Check sheet for the modelled part. Datum: model origin and axes. Units: mm. Face numbers are marked on the shaded views. A direction names the side the tool comes from. Coordinates: 2 decimals unless noted, no trailing zeros. Order: outer loops, then holes, each group sorted by start corner. A loop starts at its lowest first (then second) coordinate and runs counter-clockwise, first axis right, second up.
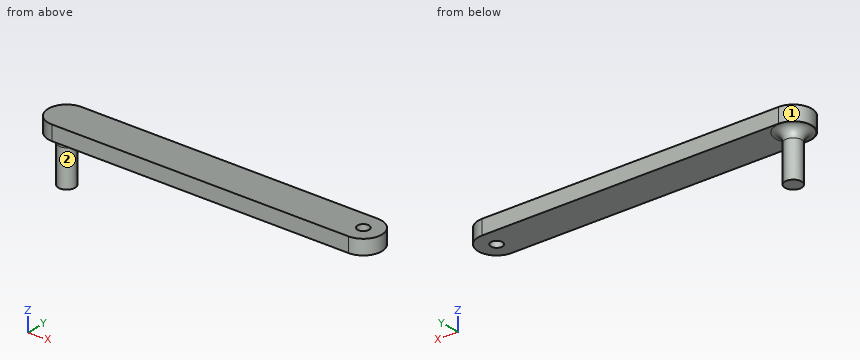
from build123d import *

# Parameters (mm, degrees)
BOSS_EXTRUDE1_DEPTH = 4
SKETCH2_R           = 2.25
BOSS_EXTRUDE2_DEPTH = 12.5
FILLET1_R           = 2.5
SKETCH4_R           = 1.575
CUT_EXTRUDE1_DEPTH  = 147.021402541


with BuildPart() as part:
    # Sketch1 → Boss-Extrude1 (new body)
    with BuildSketch(Plane.XY):
        with BuildLine():
            Line((-60, -5), (-140, -5))
            ThreePointArc((-140, -5), (-145, 0), (-140, 5))
            Line((-140, 5), (-60, 5))
            ThreePointArc((-60, 5), (-55, 0), (-60, -5))
        make_face()
    extrude(amount=BOSS_EXTRUDE1_DEPTH)

    # Sketch2 → Boss-Extrude2 (add)
    with BuildSketch(Plane(origin=(0, 0, 0), x_dir=(-1, 0, 0), z_dir=(0, 0, -1))):
        with Locations(Location((140, 0, 0), (0, 0, 180))):
            Circle(SKETCH2_R)
    extrude(amount=BOSS_EXTRUDE2_DEPTH)

    # Fillet1
    fillet1_edges = [part.edges().sort_by_distance(p)[0] for p in [
        (-142.25, 0, 0),
    ]]
    fillet(fillet1_edges, radius=FILLET1_R)

    # Sketch4 → Cut-Extrude1 (cut, through all)
    with BuildSketch(Plane.XY.offset(4)):
        with Locations((-60, 0)):
            Circle(SKETCH4_R)
    extrude(amount=-CUT_EXTRUDE1_DEPTH, mode=Mode.SUBTRACT)


solid = part.part
(1) Tool access check on the marked faces 1 and 2. Record the directions out of +Z, -Z, +X, -X, +Y, -Y that give a thin tool (end or side, any length) a straight path to the whole face; none if there is none.
Filled in:
face 1: +Z, -Z, -X
face 2: -Z
(2) Cross-section at B-B (z = 1.5). Enter the section's corners in (x, y) (3 decimals).
Filled in:
outline: (-140, -5) - (-60, -5) arc R5 ccw to (-60, 5) - (-140, 5) arc R5 ccw to start; hole circle Ø3.15 at (-60, 0)
(3) Cross-section at C-C (x = -77). Enter the section's corners in (y, z).
Filled in:
outline: (-5, 0) - (5, 0) - (5, 4) - (-5, 4) - close
(4) Go/stop test with flat-tipped pins: P1, Ø2.5, axis at x = -60, y = 0, coming from the +Z side; P2, Ø4, axis at y = 4, z = -5.5, coming from the -X side; P3, Ø5, axis at x = -109.5, y = 0.5, coming from the -Z side. Record where each tip stops, or that it passes through.
Filled in:
P1: passes through
P2: stops at x = -141.03
P3: stops at z = 0
(5) Thickness scan on probe 1 along Z at (x, y) = (-128, -0.75); probe 2 along Y at (x, z) = (-60, 1.95) (3 decimals); probe 3 along X at (y, z) = (-0.75, -1). Record the ranges inside material, lowest first.
Filled in:
probe 1: z = 0 to 4
probe 2: y = -5 to -1.575, 1.575 to 5
probe 3: x = -142.65 to -137.35
(6) Cross-section at A-A (y = 0). Enter the section's corners in (x, z) (3 decimals), and give its area (3 significant figures).
Filled in:
outline: (-145, 0) - (-144.75, 0) arc R2.5 cw to (-142.25, -2.5) - (-142.25, -12.5) - (-137.75, -12.5) - (-137.75, -2.5) arc R2.5 cw to (-135.25, 0) - (-61.575, 0) - (-61.575, 4) - (-145, 4) - close; (-58.425, 0) - (-55, 0) - (-55, 4) - (-58.425, 4) - close
area: 406 mm2
